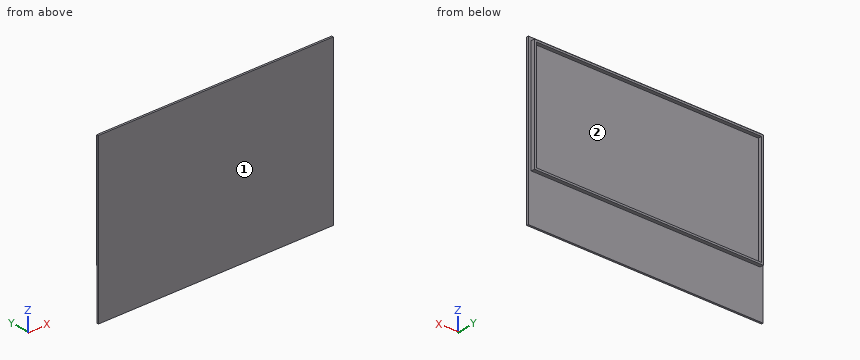
from build123d import *

# Parameters (mm, degrees)
SKETCH1_W           = 203.2
SKETCH1_H           = 101.6
BOSS_EXTRUDE1_DEPTH = 1.5875
SKETCH2_W           = 198.12
SKETCH2_H           = 96.52
BOSS_EXTRUDE2_DEPTH = 3.175
SKETCH3_W           = 194.945
SKETCH3_H           = 93.345
CUT_EXTRUDE1_DEPTH  = 3.175
SKETCH5_W           = 203.2
SKETCH5_H           = 1.5875
BOSS_EXTRUDE3_DEPTH = 38.1


with BuildPart() as part:
    # Sketch1 → Boss-Extrude1 (new body)
    with BuildSketch(Plane(origin=(0, 0, 0), x_dir=(1, 0, 0), z_dir=(0, 1, 0))):
        Rectangle(SKETCH1_W, SKETCH1_H)
    extrude(amount=BOSS_EXTRUDE1_DEPTH)

    # Sketch2 → Boss-Extrude2 (add)
    with BuildSketch(Plane(origin=(0, 1.5875, 0), x_dir=(1, 0, 0), z_dir=(0, 1, 0))):
        Rectangle(SKETCH2_W, SKETCH2_H)
    extrude(amount=BOSS_EXTRUDE2_DEPTH)

    # Sketch3 → Cut-Extrude1 (cut)
    with BuildSketch(Plane(origin=(0, 4.7625, 0), x_dir=(1, 0, 0), z_dir=(0, 1, 0))):
        Rectangle(SKETCH3_W, SKETCH3_H)
    extrude(amount=-CUT_EXTRUDE1_DEPTH, mode=Mode.SUBTRACT)

    # Sketch5 → Boss-Extrude3 (add)
    with BuildSketch(Plane(origin=(0, 0, -50.8), x_dir=(-1, 0, 0), z_dir=(0, 0, -1))):
        with Locations((0, 0.79375)):
            Rectangle(SKETCH5_W, SKETCH5_H)
    extrude(amount=BOSS_EXTRUDE3_DEPTH)


solid = part.part
Part model, mm, in its own coordinate system. Face numbers are marked on the shaded views. Coordinates: 2 decimals unless noted, no trailing zeros. Order: outer loops, then holes, each group sorted by start corner. A loop starts at its lowest first (then second) coordinate and runs counter-clockwise, first axis right, second up. Notation, with made-up numbers: (85, 25) - (117, 25) arc R10 ccw to (117, 30) - close; hole circle Ø9 at (19.25, 21.25). An arc over 180 degrees is marked (long way). Use CSV: the item, a comma, the result in double quotes.
Item 1: Probe probe 1 along Z at (x, y) = (-58, 2.85); probe 2 along X at (y, z) = (2.75, -25.5); probe 3 along Y at (x, z) = (32, 23.5). List the from-to ranges inside material, lowest first.
Solved:
probe 1,"z = -48.26 to -46.67, 46.67 to 48.26"
probe 2,"x = -99.06 to -97.47, 97.47 to 99.06"
probe 3,"y = 0 to 1.59"
Item 2: Drop flat-ended pins along their axis: P1, Ø1, axis at y = 3, z = 19.5, coming from the -X side; P2, Ø2.5, axis at y = 3, z = -21, coming from the +X side; P3, Ø1.6, axis at x = -12.5, y = 3.5, coming from the +Z side; P4, Ø1.5, axis at y = 2.5, z = -63, coming from the -X side. Give the stop position or say it passes through.
Solved:
P1,"stops at x = -99.06"
P2,"stops at x = 99.06"
P3,"stops at z = 48.26"
P4,"passes through"
Item 3: Mould opens along X. For the marked faces 1 and 2 say: +X half, -X half, draft (parallel to the pull), parting line (faces both ways), or undercut.
Solved:
face 1,"draft"
face 2,"undercut"
Item 4: Saw through at D-D on z = -78. Give the cut face in (x, y), and give its area (3 significant figures).
Solved:
outline,"(-101.6, 0) - (101.6, 0) - (101.6, 1.59) - (-101.6, 1.59) - close"
area,"323 mm²"
Item 5: Saw through at B-B on z = -38. Give the cut face in (x, y), and give its area (3 significant figures).
Solved:
outline,"(-101.6, 0) - (101.6, 0) - (101.6, 1.59) - (99.06, 1.59) - (99.06, 4.76) - (97.47, 4.76) - (97.47, 1.59) - (-97.47, 1.59) - (-97.47, 4.76) - (-99.06, 4.76) - (-99.06, 1.59) - (-101.6, 1.59) - close"
area,"333 mm²"
Item 6: Saw through at A-A on y = 2.6. Give the cut face in (x, z).
Solved:
outline,"(-99.06, -48.26) - (99.06, -48.26) - (99.06, 48.26) - (-99.06, 48.26) - close; hole (-97.47, -46.67) - (97.47, -46.67) - (97.47, 46.67) - (-97.47, 46.67) - close"
Item 7: Saw through at C-C on x = 52.5. Give the cut face in (y, z).
Solved:
outline,"(0, -88.9) - (1.59, -88.9) - (1.59, -48.26) - (4.76, -48.26) - (4.76, -46.67) - (1.59, -46.67) - (1.59, 46.67) - (4.76, 46.67) - (4.76, 48.26) - (1.59, 48.26) - (1.59, 50.8) - (0, 50.8) - close"
